Could you check a few things on this model? Use its own coordinates, in mm. Face numbers are marked on the shaded views. Give positions to 0.01 mm unless a question says otherwise; leave off trailing zeros. Write each question's results on one line, items separated by ' | '.
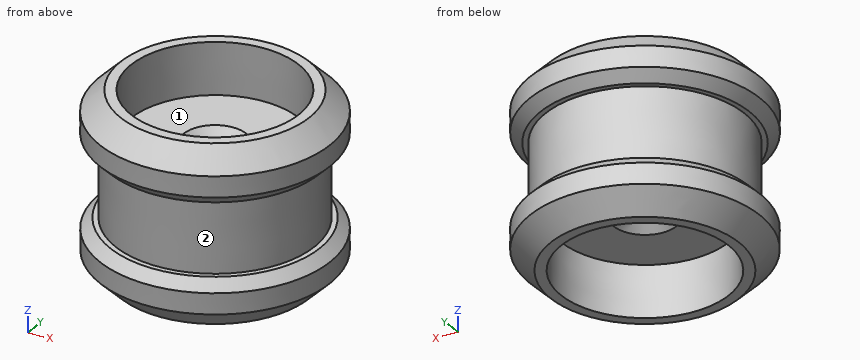
```python
from build123d import *

# Parameters (mm, degrees)
F2_SIZE = 2
F3_SIZE = 1


with BuildPart() as f1:
    # F0 (on Front) → F1 (revolve)
    with BuildSketch(Plane.XZ):
        Polygon((11.0896060326, 2.2645946667), (8.0896060326, 2.2645946667), (8.0896060326, -2.7354053333), (9.5896060326, -2.7354053333), (11.0896060326, -2.7354053333), align=None)
        Polygon((9.5896060326, -2.7354053333), (8.0896060326, -2.7354053333), (1.9999996262, -2.7354053333), (1.9999996262, -9.7354053333), (8.0896060326, -9.7354053333), (9.5896060326, -9.7354053333), (9.5896060326, -2.7403513981), align=None)
        Polygon((11.0896060326, -9.7354053333), (9.5896060326, -9.7354053333), (8.0896060326, -9.7354053333), (8.0896060326, -14.7354053333), (11.0896060326, -14.7354053333), align=None)
    revolve(axis=Axis((-0.0051969837, 0, -6.2354053333), (0.0006114097, 0, -0.9999998131)))

    # F2
    f2_edges = [f1.edges().sort_by_distance(p)[0] for p in [
        (-11.089598, 0, -14.748966),
        (-11.110386, 0, 2.251021),
    ]]
    chamfer(f2_edges, length=F2_SIZE)

    # F3
    f3_edges = [f1.edges().sort_by_distance(p)[0] for p in [
        (-11.104272, 0, -2.748975),
        (-11.095712, 0, -9.74897),
        (-2.014672, 0, -2.73786),
        (-2.006112, 0, -9.737855),
    ]]
    chamfer(f3_edges, length=F3_SIZE)


solid = f1.part
```
Q1. I need wall thicknesses on line 1 along Z through (x, y) = (-3.5, 5.75); line 2 along Y through (x, z) = (-1.5, -4); line 3 along Z through (x, y) = (-6, -6.75). Which ranges of each line are inside material? Lowest first, please.
Here are the results:
line 1: z = -9.74 to -2.74 | line 2: y = -9.48 to -1.34, 1.34 to 9.48 | line 3: z = -14.74 to 2.26
Q2. Thinking about a two-plate mould opening in Z: for the marked faces 1 and 2, which applies, +Z half, -Z half, draft (parallel to the pull), parting line (faces both ways), or undercut?
Here are the results:
face 1: +Z half | face 2: undercut
Q3. I'm going to push flat-ended pins straight in: pin 1 Ø3 at (x, y) = (-4, 8) entering from +Z; pin 2 Ø6 at (y, z) = (2, -5) entering from +X; pin 3 Ø1 at (y, z) = (-3, -6) entering from -X. Where does each tip first touch, or does it pass through?
Here are the results:
pin 1: stops at z = 2.26 | pin 2: stops at x = 10.68 | pin 3: stops at x = -9.27
